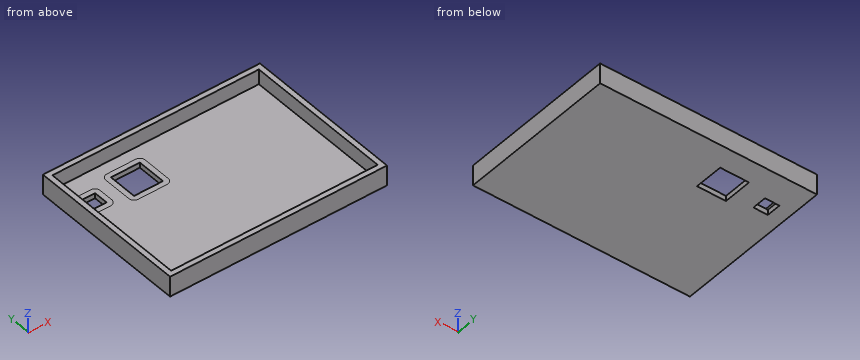
```python
from build123d import *

# Parameters (mm, degrees)
F0_W     = 75
F0_H     = 55
F0_W_2   = 5
F0_H_2   = 5
F0_W_3   = 10
F0_H_3   = 10
F1_DEPTH = 7
F2_T     = -1.8
F3_W     = 35
F3_H     = 9.282675
F4_DEPTH = 25


with BuildPart() as f1:
    # F0 (on Top) → F1 (new body)
    with BuildSketch(Plane.XY):
        Rectangle(F0_W, F0_H)
        with Locations((-30, 15)):
            Rectangle(F0_W_2, F0_H_2, mode=Mode.SUBTRACT)
        with Locations((-15, 15)):
            Rectangle(F0_W_3, F0_H_3, mode=Mode.SUBTRACT)
    extrude(amount=F1_DEPTH)

    # F2
    f2_openings = [f1.faces().sort_by_distance(p)[0] for p in [
        (0.5625, -0.46875, 7),
    ]]
    offset(amount=F2_T, openings=f2_openings)

    # F3 (on Front) → F4 (cut)
    with BuildSketch(Plane.XZ):
        with Locations((-17.5, 6.441337)):
            Rectangle(F3_W, F3_H)
    extrude(amount=-F4_DEPTH, mode=Mode.SUBTRACT)


solid = f1.part
```
For this review, take the finished solid that the model builds, in its own axes (mm). Round coordinates to 2 decimals unless told otherwise and drop trailing zeros. Loops run counter-clockwise (first coordinate to the right, second up) from the corner with the lowest first, then second, coordinate; pieces in that order, holes last.
Q1. Insertion check: pin 1 Ø8 at (x, y) = (-21.5, 13.5) entering from +Z. The pin has a flat end and moves straight along its axis. Give the tip position at first contact, or say it passes through.
Result sheet:
pin 1: stops at z = 1.8
Q2. Add section A-A on z = 3.5. Write out the cut boundary in (x, y), plus the area to 3 significant figures.
Result sheet:
outline: (-37.5, -27.5) - (37.5, -27.5) - (37.5, 27.5) - (-37.5, 27.5) - close; hole (-35.7, -25.7) - (35.7, -25.7) - (35.7, 25.7) - (-35.7, 25.7) - close
area: 455 mm2
Q3. Add section B-B on y = 15.5. Write out the cut boundary in (x, z), plus the area to 3 significant figures.
Result sheet:
outline: (-37.5, 0) - (-32.5, 0) - (-32.5, 1.8) - (-35.7, 1.8) - (-35.7, 7) - (-37.5, 7) - close; (-27.5, 0) - (-20, 0) - (-20, 1.8) - (-27.5, 1.8) - close; (-10, 0) - (37.5, 0) - (37.5, 7) - (35.7, 7) - (35.7, 1.8) - (-10, 1.8) - close
area: 127 mm2
Q4. To check wall thickness, follow line 1 along X through (y, z) = (14, 0.75); line 2 along X through (y, z) = (-9, 3.25); line 3 along Y through (x, z) = (11, 2.5). State the ranges of each line that lie inside material, in increasing order.
Result sheet:
line 1: x = -37.5 to -32.5, -27.5 to -20, -10 to 37.5
line 2: x = -37.5 to -35.7, 35.7 to 37.5
line 3: y = -27.5 to -25.7, 25.7 to 27.5
Q5. Add section C-C on x = 3.5. Write out the cut boundary in (y, z), plus the area to 3 significant figures.
Result sheet:
outline: (-27.5, 0) - (27.5, 0) - (27.5, 7) - (25.7, 7) - (25.7, 1.8) - (-25.7, 1.8) - (-25.7, 7) - (-27.5, 7) - close
area: 118 mm2
Q6. Add section D-D on y = -17. Write out the cut boundary in (x, z).
Result sheet:
outline: (-37.5, 0) - (37.5, 0) - (37.5, 7) - (35.7, 7) - (35.7, 1.8) - (-35.7, 1.8) - (-35.7, 7) - (-37.5, 7) - close
